Can you work these out from the model? Positions are in its coordinate system, mm. A direction names the side the tool comes from. Give positions to 0.01 mm unless a question says otherwise; leave off trailing zeros. Write each loop counter-clockwise with the first axis right and the second up, starting at its lowest first coordinate (ties: lowest second). Pieces come first, ordered by that corner, then holes. Notation, with made-up numbers: M -11,46.5 L 42,46.5 A10 cw 42,62.5 Z; hole C -33.75,38.5 d6. An arc over 180 degrees is marked long. Write each question's results on one line, items separated by ' | '.
from build123d import *

# Parameters (mm, degrees)
SKETCH1_W           = 97.028
SKETCH1_H           = 22.352
SKETCH1_R           = 1.5875
BOSS_EXTRUDE1_DEPTH = 1.524
SKETCH1_3_W         = 41.402
SKETCH1_3_H         = 22.352
BOSS_EXTRUDE2_DEPTH = 15.748


with BuildPart() as part:
    # Sketch1 → Boss-Extrude1 (new body)
    with BuildSketch(Plane(origin=(0, 0, 0), x_dir=(1, 0, 0), z_dir=(0, 1, 0))):
        with Locations((22.805106227, 0)):
            Rectangle(SKETCH1_W, SKETCH1_H)
        with Locations((-22.089393773, 0)):
            Circle(SKETCH1_R, mode=Mode.SUBTRACT)
        with Locations((67.699606227, 0)):
            Circle(SKETCH1_R, mode=Mode.SUBTRACT)
    extrude(amount=BOSS_EXTRUDE1_DEPTH)

    # Sketch1_3 → Boss-Extrude2 (add)
    with BuildSketch(Plane(origin=(0, 0, 0), x_dir=(1, 0, 0), z_dir=(0, 1, 0))):
        with Locations((2.104106227, 0)):
            Rectangle(SKETCH1_3_W, SKETCH1_3_H)
        with Locations((43.506106227, 0)):
            Rectangle(SKETCH1_3_W, SKETCH1_3_H)
    extrude(amount=BOSS_EXTRUDE2_DEPTH)


solid = part.part
Item 1: If I drill on line 1 (X direction, y = 0.8, z = 0); line 2 (X direction, y = 6.75, z = 8.5), over which ranges is the centre line in solid material (lowest first)? Write a range as from..to.
Geometry says:
line 1: x = -25.71..-23.68, -20.5..66.11, 69.29..71.32 | line 2: x = -18.6..64.21
Item 2: I want a section at C-C, the plane y = 8. Please give me the cut outline in (x, z).
Geometry says:
outline: M -18.6,-11.18 L 64.21,-11.18 L 64.21,11.18 L -18.6,11.18 Z
Item 3: I want a section at A-A, the plane z = 0. Please give me the cut outline in (x, y), and give its area (3 significant figures).
Geometry says:
outline: M -25.71,0 L -23.68,0 L -23.68,1.52 L -25.71,1.52 Z; M -20.5,0 L 66.11,0 L 66.11,1.52 L 64.21,1.52 L 64.21,15.75 L -18.6,15.75 L -18.6,1.52 L -20.5,1.52 Z; M 69.29,0 L 71.32,0 L 71.32,1.52 L 69.29,1.52 Z | area: 1,320 mm2
Item 4: I'm going to push flat-ended pins straight in: pin 1 (1.9 mm diameter, centred on x = 67.7, z = 0, fed in from +Y); pin 2 (6 mm diameter, centred on y = 9, z = 3.5, fed in from -X); pin 3 (8 mm diameter, centred on x = -24, z = 5, fed in from +Y); pin 4 (4.5 mm diameter, centred on y = 10.5, z = -5, fed in from +X). Where does each tip first touch, or does it pass through?
Geometry says:
pin 1: passes through | pin 2: stops at x = -18.6 | pin 3: stops at y = 1.52 | pin 4: stops at x = 64.21
Item 5: Thinking about a two-plate mould opening in Z: for faces 4 (the face through (22, 8, 11.176)), 5 (the face through (-20.575, 0.751, -0.477)), 6 (the face through (-25.709, 1, 0)), which applies, +Z half, -Z half, draft (parallel to the pull), parting line (faces both ways), or undercut?
Geometry says:
face 4: +Z half | face 5: undercut | face 6: draft
Item 6: I want a section at B-B, the plane z = -6.25. Please give me the cut outline in (x, y).
Geometry says:
outline: M -25.71,0 L 71.32,0 L 71.32,1.52 L 64.21,1.52 L 64.21,15.75 L -18.6,15.75 L -18.6,1.52 L -25.71,1.52 Z
Item 7: For faces 1 (the face through (-18.597, 9, 0)), 2 (the face through (66.53, 0.751, -1.073)), 3 (the face through (64.207, 9, 0)), which set-ups out of +Z, -Z, +X, -X, +Y, -Y let a thin tool reach every point of the face, with its end or its side?
Geometry says:
face 1: +Z, -Z, -X, +Y | face 2: +Y, -Y | face 3: +Z, -Z, +X, +Y
